For this review, use the dimensioned drawing (mm, ordinates from the lowest corner) and the shaded views. A direction names the side the tool comes from. Give positions to 0.01 mm unless a question says otherwise; leave off trailing zeros. Order: outer loops, then holes, each group sorted by start corner. A loop starts at its lowest first (then second) coordinate and runs counter-clockwise, first axis right, second up. Notation, with made-up numbers: (36, 34.5) - (91, 34.5) arc R16 cw to (91, 50.5) - close; hole circle Ø11 at (86, 4.5). An arc over 180 degrees is marked (long way). One line per item, written item: value.
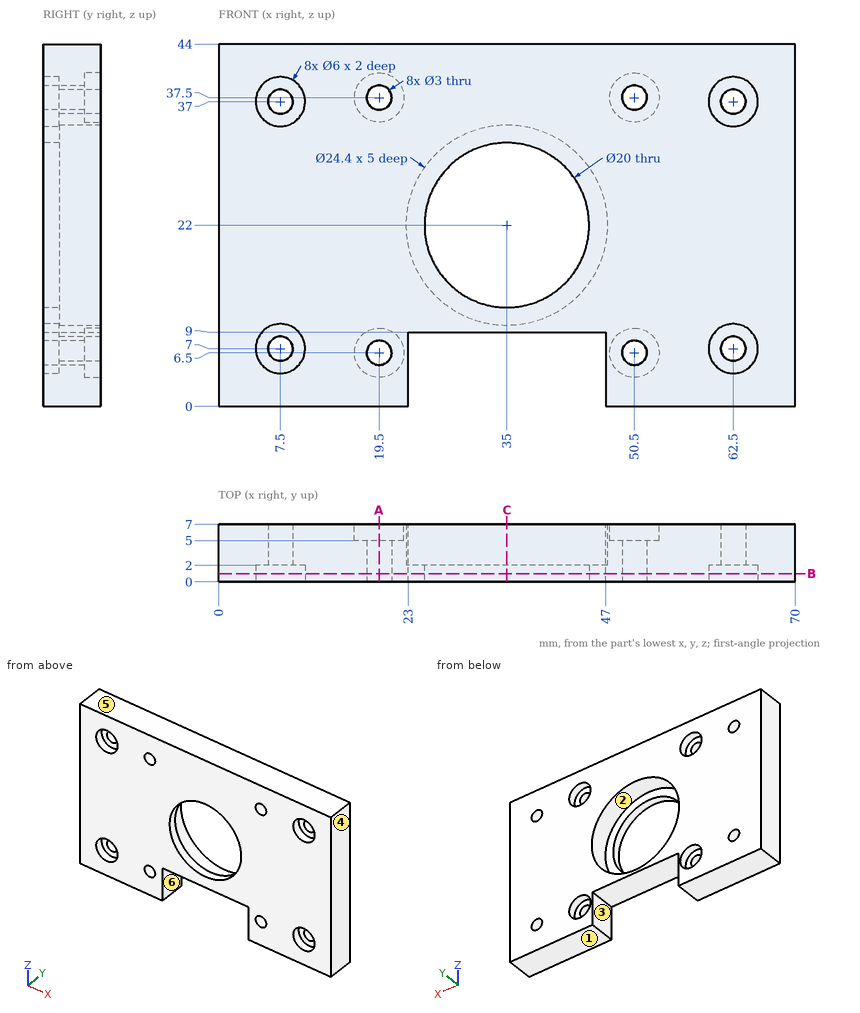
(1) Take a section at C-C (x = 35). Write out the cut boundary in (y, z).
Answers below:
outline: (0, 9) - (7, 9) - (7, 9.8) - (2, 9.8) - (2, 12) - (0, 12) - close; (0, 32) - (2, 32) - (2, 34.2) - (7, 34.2) - (7, 44) - (0, 44) - close
(2) Wall thickness on line 1 (Z direction, x = 7.5, y = 6); line 2 (Z direction, x = 50.5, y = 2.1); line 3 (X direction, y = 2.6, z = 6.5): over which ranges is each line inside the solid? List them lowest first. Write a range as from..to.
Answers below:
line 1: z = 0..5.5, 8.5..35.5, 38.5..44
line 2: z = 0..5, 8..36, 39..44
line 3: x = 0..6.09, 8.91..18, 21..23, 47..49, 52..61.09, 63.91..70
(3) Machinability: for the marked faces 1, 2 and 3, which of the approach directions +Z, -Z, +X, -X, +Y, -Y give a long, thin tool a straight path to every point of the face, cutting with its end or side? Answer none if there is none.
Answers below:
face 1: -Z, +X, -X, +Y, -Y
face 2: +Y
face 3: -Z, +Y, -Y
(4) Take a section at A-A (x = 19.5). Write out the cut boundary in (y, z).
Answers below:
outline: (0, 0) - (7, 0) - (7, 3.5) - (5, 3.5) - (5, 5) - (0, 5) - close; (0, 8) - (5, 8) - (5, 9.5) - (7, 9.5) - (7, 34.5) - (5, 34.5) - (5, 36) - (0, 36) - close; (0, 39) - (5, 39) - (5, 40.5) - (7, 40.5) - (7, 44) - (0, 44) - close
(5) Take a section at B-B (y = 1). Give the number of separate pieces and of enclosed holes in the cut face, then the cut area to 3 significant figures.
Answers below:
separate pieces: 1
enclosed holes: 9
area: 2,410 mm^2
(6) For P1, Ø1.5, axis at x = 36, z = 14.5, coming from the +Y side; P2, Ø3, axis at x = 38, y = 1, coming from the -Z side; P3, Ø1.8, axis at x = 63.5, z = 7.5, coming from the -Y side; P4, Ø5, axis at x = 50.5, z = 37.5, coming from the +Y side, all flat-tipped, find the tip position at first contact; note any pin that passes through.
Answers below:
P1: passes through
P2: stops at z = 9
P3: stops at y = 2
P4: stops at y = 5
(7) Draft analysis for pull direction X (two halves, no side actions). For the marked faces 4, 5 and 6, state which applies: pulls with the +X half, pulls with the -X half, needs draft (parallel to the pull), parting line crosses it, or undercut.
Answers below:
face 4: pulls with the +X half
face 5: needs draft
face 6: undercut
